```python
from build123d import *

# Parameters (mm, degrees)
PAD_DEPTH          = 8
SKETCH001_W        = 12.2
SKETCH001_H        = 8.2
POCKET_DEPTH       = 8
POLARPATTERN_COUNT = 3


with BuildPart() as part:
    # Sketch → Pad (new body)
    with BuildSketch(Plane.XY):
        with BuildLine():
            ThreePointArc((-29.53026, 52.229912), (0, -60), (29.53026, 52.229912))
            Line((29.53026, 122.229912), (29.53026, 52.229912))
            Line((23.53026, 122.229912), (29.53026, 122.229912))
            Line((23.53026, 122.229912), (23.53026, 82.229912))
            Line((23.53026, 82.229912), (-29.53026, 52.229912))
        make_face()
    extrude(amount=PAD_DEPTH)

    # Sketch001 → Pocket (cut)
    with BuildSketch(Plane.XY.offset(8)):
        with Locations((0, -35.432139)):
            Rectangle(SKETCH001_W, SKETCH001_H)
    pocket = extrude(amount=-POCKET_DEPTH, mode=Mode.SUBTRACT)

    # PolarPattern: Pocket ×3 about axis
    polarpattern_axis = Axis((0, 0, 8), (0, 0, 1))
    for i in range(1, POLARPATTERN_COUNT):
        add(pocket.rotate(polarpattern_axis, i * 360 / POLARPATTERN_COUNT), mode=Mode.SUBTRACT)


solid = part.part
```
Part model, mm, in its own coordinate system. A direction names the side the tool comes from. Round coordinates to 2 decimals unless told otherwise and drop trailing zeros. Loops run counter-clockwise (first coordinate to the right, second up) from the corner with the lowest first, then second, coordinate; pieces in that order, holes last.
Item 1: Cut at B-B, the plane x = 0. Give the cut face in (y, z).
Item 2: Drill centre lines: line 1 (X direction, y = 15, z = 1.5); line 2 (X direction, y = 109, z = 5); line 3 (X direction, y = 0, z = 1). Where is each one in solid material? Low to high.
Item 3: Mould opens along X. For faces 4 (the face through (-27.09, 15.74, 4.06)), 5 (the face through (23.53, 103, 4)), 6 (the face through (-1, 12, 8)) say: +X half, -X half, draft (parallel to the pull), parting line (faces both ways), or undercut.
Item 4: 3-axis set-ups, long thin cutter, end or side, ignore diameter. For faces 1 (the face through (29.53, 88, 4)), 2 (the face through (-1, 12, 0)), 3 (the face through (27.685, 23.028, 4.056)): which of +Z, -Z, +X, -X, +Y, -Y reach the whole face in a straight line?
Item 5: Drop flat-ended pins along their axis: P1, Ø4, axis at x = 11, z = 1.5, coming from the +Y side; P2, Ø3, axis at y = 48.5, z = 2, coming from the -X side; P3, Ø4, axis at y = -37, z = 5.5, coming from the -X side. Give the stop position or say it passes through.
Item 6: Cut at C-C, the plane y = -23.5. Give the cut face in (x, z), then the cut area to 3 significant figures.
Item 7: Cut at A-A, the plane z = 4. Give the cut face in (x, y).
Item 8: Cut at D-D, the plane x = 17.5. Give the cut face in (y, z), then the cut area to 3 significant figures.
A:
1. outline: (-60, 0) - (-39.53, 0) - (-39.53, 8) - (-60, 8) - close; (-31.33, 0) - (68.93, 0) - (68.93, 8) - (-31.33, 8) - close
2. line 1: x = -58.09 to -36.99, -27.52 to 27.52, 36.99 to 58.09
2. line 2: x = 23.53 to 29.53
2. line 3: x = -60 to 60
3. face 4: undercut
3. face 5: -X half
3. face 6: draft
4. face 1: +Z, -Z, +X, +Y
4. face 2: -Z, +X, -X, +Y, -Y
4. face 3: +Z, -Z
5. P1: stops at y = 76.28
5. P2: stops at x = -37.3
5. P3: stops at x = -48.73
6. outline: (-55.21, 0) - (55.21, 0) - (55.21, 8) - (-55.21, 8) - close
6. area: 883 mm2
7. outline: (-29.53, 52.23) arc R60 ccw (long way) to (29.53, 52.23) - (29.53, 122.23) - (23.53, 122.23) - (23.53, 82.23) - close; hole (-37.29, 14.48) - (-30.18, 10.38) - (-24.08, 20.95) - (-31.19, 25.05) - close; hole (-6.1, -39.53) - (6.1, -39.53) - (6.1, -31.33) - (-6.1, -31.33) - close; hole (24.08, 20.95) - (30.18, 10.38) - (37.29, 14.48) - (31.19, 25.05) - close
8. outline: (-57.39, 0) - (78.82, 0) - (78.82, 8) - (-57.39, 8) - close
8. area: 1,090 mm2
